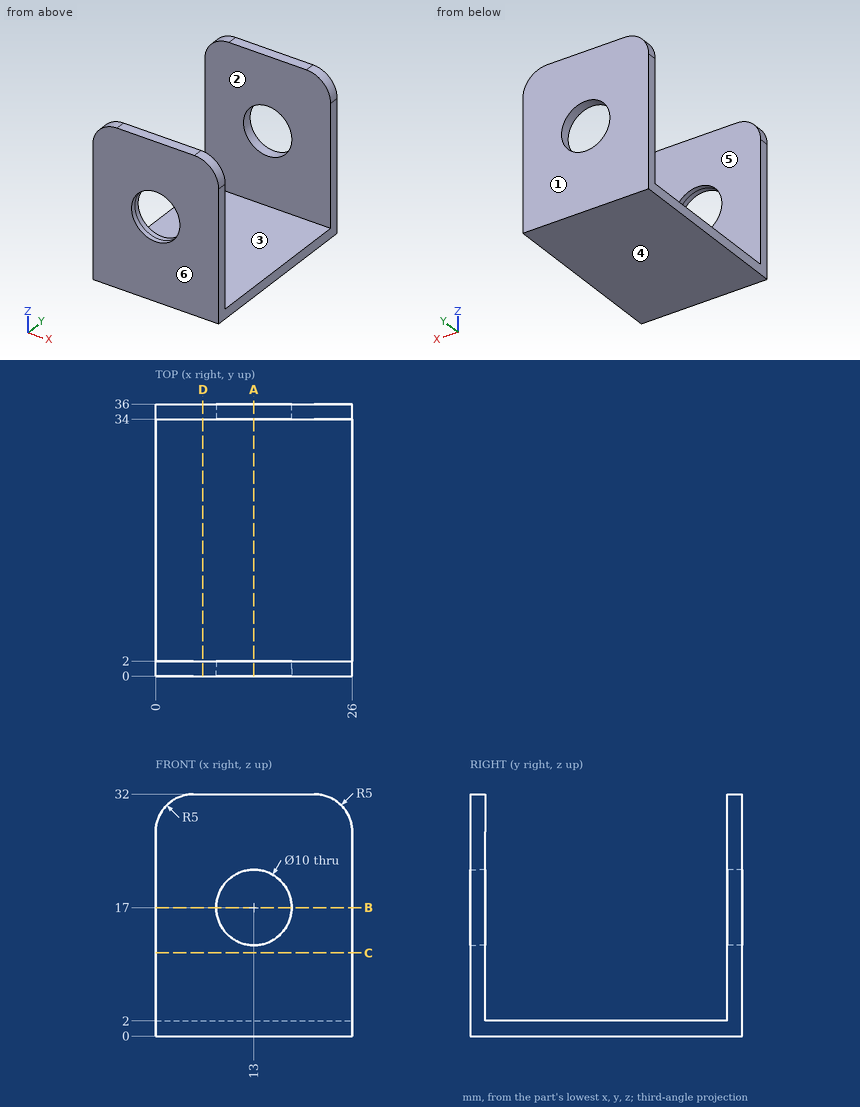
For this review, use the dimensioned drawing (mm, ordinates from the lowest corner) and the shaded views. A direction names the side the tool comes from. Coordinates: 2 decimals unless noted, no trailing zeros. Loops run counter-clockwise (first coordinate to the right, second up) from the corner with the lowest first, then second, coordinate; pieces in that order, holes last. Notation, with made-up numbers: (-5, 44) -> (34, 44) arc R26 ccw to (34, 74) -> close; hole circle Ø4 at (68.25, 3). An arc over 180 degrees is marked (long way). Use a Markdown table: item, result. Add a question column.
Item 1: Clearance check with flat-ended pins moving along their axes: P1, Ø8, axis at x = 13, z = 17, coming from the +Y side; P2, Ø13, axis at x = 13.5, y = 16.5, coming from the +Z side. State where each tip first meets the part, or that it passes through.
Item 2: Wall thickness on L1, parallel to X at y = 0.7, z = 17; L2, parallel to Y at x = 10.75, z = 26; L3, parallel to Z at x = 13, y = 35.3: over which ranges is each line inside the solid? List them lowest first. Write a range as from..to.
Item 3: We need section A-A, the plane x = 13. Write out the cut boundary in (y, z), and give its area (3 significant figures).
Item 4: The part is to be moulded in two halves that separate along Y. For the marked faces 3, 4, 5 and 6, say which applies: +Y half, -Y half, draft (parallel to the pull), parting line (faces both ways), or undercut.
Item 5: Machinability: for the marked faces 1 and 2, which of the approach directions +Z, -Z, +X, -X, +Y, -Y give a long, thin tool a straight path to every point of the face, cutting with its end or side? Answer none if there is none.
Item 6: We need section D-D, the plane x = 6.25. Write out the cut boundary in (y, z).
Item 7: We need section B-B, the plane z = 17. Write out the cut boundary in (x, y).
Item 8: We need section C-C, the plane z = 11. Write out the cut boundary in (x, y).
Numbers:
| question | item | result |
|---|---|---|
| 1 | P1 | passes through |
| 1 | P2 | stops at z = 2 |
| 2 | L1 | x = 0..8, 18..26 |
| 2 | L2 | y = 0..2, 34..36 |
| 2 | L3 | z = 0..12, 22..32 |
| 3 | outline | (0, 0) -> (36, 0) -> (36, 12) -> (34, 12) -> (34, 2) -> (2, 2) -> (2, 12) -> (0, 12) -> close; (0, 22) -> (2, 22) -> (2, 32) -> (0, 32) -> close; (34, 22) -> (36, 22) -> (36, 32) -> (34, 32) -> close |
| 3 | area | 152 mm^2 |
| 4 | face 3 | undercut |
| 4 | face 4 | draft |
| 4 | face 5 | undercut |
| 4 | face 6 | -Y half |
| 5 | face 1 | +Z, -Z, +X, -X, +Y |
| 5 | face 2 | +Z, +X, -X |
| 6 | outline | (0, 0) -> (36, 0) -> (36, 32) -> (34, 32) -> (34, 2) -> (2, 2) -> (2, 32) -> (0, 32) -> close |
| 7 | outline | (0, 0) -> (8, 0) -> (8, 2) -> (0, 2) -> close; (0, 34) -> (8, 34) -> (8, 36) -> (0, 36) -> close; (18, 0) -> (26, 0) -> (26, 2) -> (18, 2) -> close; (18, 34) -> (26, 34) -> (26, 36) -> (18, 36) -> close |
| 8 | outline | (0, 0) -> (26, 0) -> (26, 2) -> (0, 2) -> close; (0, 34) -> (26, 34) -> (26, 36) -> (0, 36) -> close |
